Drawing for the job (mm, zero at the part's lowest x, y, z). A direction names the side the tool comes from. Give positions to 0.01 mm unless a question says otherwise; leave off trailing zeros. Order: outer loops, then holes, each group sorted by start corner. A loop starts at its lowest first (then second) coordinate and runs counter-clockwise, first axis right, second up. Notation, with made-up numbers: (52, -14) - (97, -14) arc R29 cw to (97, 22) - close; hole circle Ø4 at (34, 87). An arc over 180 degrees is marked (long way). Use a Markdown table: item, result.
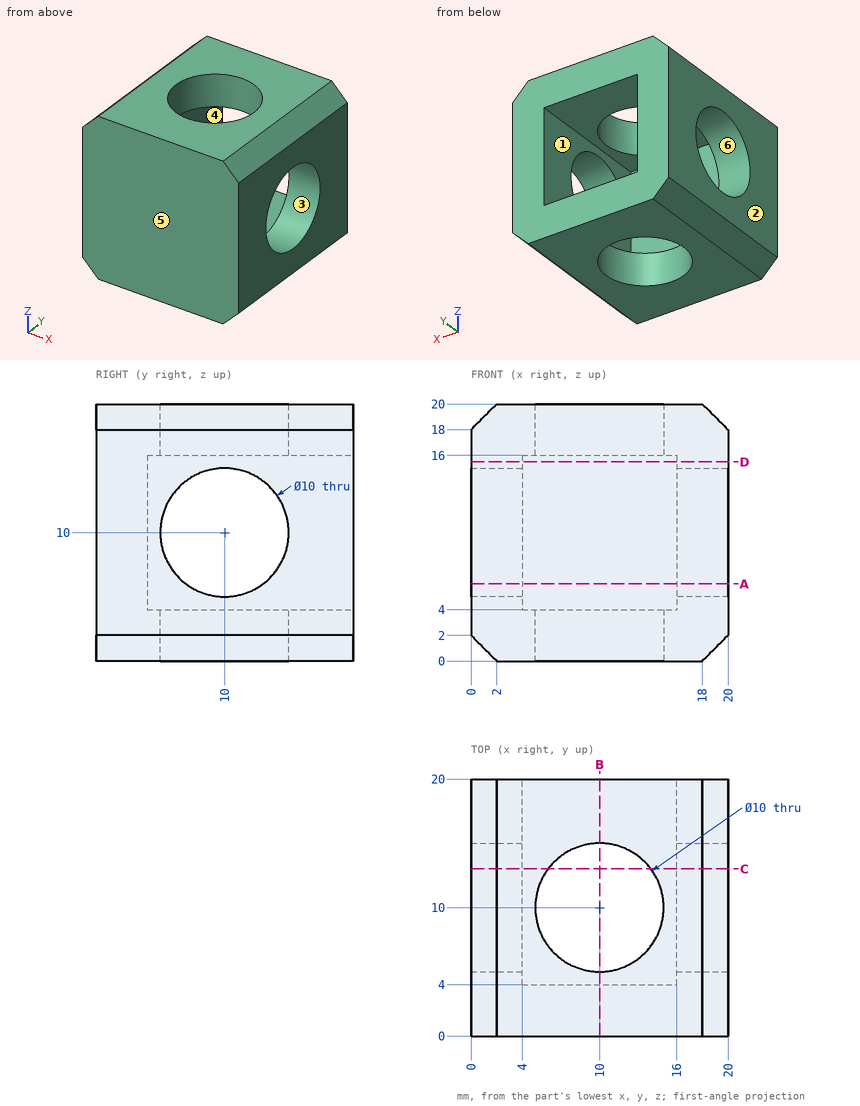
1) Slice it at C-C (y = 13). Write the cut outline in (x, z), and give its area (3 significant figures).
Computed:
| item | result |
|---|---|
| outline | (0, 2) - (2, 0) - (6, 0) - (6, 4) - (4, 4) - (4, 6) - (0, 6) - close; (0, 14) - (4, 14) - (4, 16) - (6, 16) - (6, 20) - (2, 20) - (0, 18) - close; (14, 0) - (18, 0) - (20, 2) - (20, 6) - (16, 6) - (16, 4) - (14, 4) - close; (14, 16) - (16, 16) - (16, 14) - (20, 14) - (20, 18) - (18, 20) - (14, 20) - close |
| area | 120 mm² |
2) Tool access for the marked faces 1 and 2: list every direction of +Z, -Z, +X, -X, +Y, -Y with a clear straight run to the whole face (end or side of a thin tool).
Computed:
| item | result |
|---|---|
| face 1 | +Y |
| face 2 | +Z, -Z, -X, +Y, -Y |
3) Wall check: line 1 (Y direction, x = 10.25, z = 19.25); line 2 (X direction, y = 6.5, z = 14.5). Give the ranges that are in metal, low to high. Write a range as from..to.
Computed:
| item | result |
|---|---|
| line 1 | y = 0..5.01, 14.99..20 |
| line 2 | x = 0..4, 16..20 |
4) Pin check, flat tips, straight feed: P1, Ø9.5, axis at x = 7, y = 10, coming from the -Z side; P2, Ø1, axis at x = 10, z = 15, coming from the +Y side. Stop position of each tip, or through.
Computed:
| item | result |
|---|---|
| P1 | stops at z = 0 |
| P2 | stops at y = 4 |
5) Slice it at D-D (z = 15.5). Write the cut outline in (x, y).
Computed:
| item | result |
|---|---|
| outline | (0, 0) - (20, 0) - (20, 20) - (16, 20) - (16, 4) - (4, 4) - (4, 20) - (0, 20) - close |
6) Two-plate mould, pull along Y, no slides. Class the marked faces 3, 4, 5 and 6: +Y half, -Y half, draft (parallel to the pull), parting line (faces both ways), or undercut.
Computed:
| item | result |
|---|---|
| face 3 | undercut |
| face 4 | draft |
| face 5 | -Y half |
| face 6 | undercut |
7) Slice it at A-A (z = 6). Write the cut outline in (x, y), and give its area (3 significant figures).
Computed:
| item | result |
|---|---|
| outline | (0, 0) - (20, 0) - (20, 7) - (16, 7) - (16, 4) - (4, 4) - (4, 7) - (0, 7) - close; (0, 13) - (4, 13) - (4, 20) - (0, 20) - close; (16, 13) - (20, 13) - (20, 20) - (16, 20) - close |
| area | 160 mm² |
8) Slice it at B-B (x = 10). Write the cut outline in (y, z).
Computed:
| item | result |
|---|---|
| outline | (0, 0) - (5, 0) - (5, 4) - (4, 4) - (4, 16) - (5, 16) - (5, 20) - (0, 20) - close; (15, 0) - (20, 0) - (20, 4) - (15, 4) - close; (15, 16) - (20, 16) - (20, 20) - (15, 20) - close |
